from build123d import *

# Parameters (mm, degrees)
F1_DEPTH = 50
F1_TAPER = -3
F2_R     = 35
F3_SIZE  = 10
F5_DEPTH = 10


with BuildPart() as f1:
    # F0 (on Top) → F1 (new body)
    with BuildSketch(Plane.XY):
        with BuildLine():
            ThreePointArc((150, -150), (300, 0), (150, 150))
            Line((150, 150), (-150, 150))
            ThreePointArc((-150, 150), (-300, 0), (-150, -150))
            Line((-150, -150), (150, -150))
        make_face()
    extrude(amount=F1_DEPTH, taper=F1_TAPER)

    # F2
    f2_edges = [f1.edges().sort_by_distance(p)[0] for p in [
        (-302.620389, 0, 50),
        (0, -152.620389, 50),
        (302.620389, 0, 50),
        (0, 152.620389, 50),
    ]]
    fillet(f2_edges, radius=F2_R)

    # F3
    f3_edges = [f1.edges().sort_by_distance(p)[0] for p in [
        (-300, 0, 0),
        (0, -150, 0),
        (300, 0, 0),
        (0, 150, 0),
    ]]
    chamfer(f3_edges, length=F3_SIZE)

    # F4 (on face) → F5 (join)
    with BuildSketch(Plane(origin=(0, 0, 0), x_dir=(1, 0, 0), z_dir=(0, 0, -1))):
        with BuildLine():
            Line((150, 128), (-150, 128))
            ThreePointArc((-150, 128), (-278, 0), (-150, -128))
            Line((-150, -128), (150, -128))
            ThreePointArc((150, -128), (278, 0), (150, 128))
        make_face()
    extrude(amount=F5_DEPTH)


solid = f1.part
Read the model definition and answer for the solid it produces. Units are mm, in the model's axes. A direction names the side the tool comes from. Give positions to 0.01 mm unless a question says otherwise; leave off trailing zeros. Loops run counter-clockwise (first coordinate to the right, second up) from the corner with the lowest first, then second, coordinate; pieces in that order, holes last. Notation, with made-up numbers: (39.25, 64.5) - (65.25, 64.5) arc R9 ccw to (65.25, 81.5) - close; hole circle Ø5 at (74.25, -5). An arc over 180 degrees is marked (long way). Answer as CSV lines item,"result". Start each with the question number.
1) Find section B-B (z = 27.5). Write down the section's boundary in (x, y), then the cut area to 3 significant figures.
2) Find section A-A (x = 100). Write down the section's boundary in (y, z), then the cut area to 3 significant figures.
3) Which of the six approach directions +Z, -Z, +X, -X, +Y, -Y give full straight-line access (tool end or side, diameter ignored) to faces 1 (the face through (1, -134, 0)), 2 (the face through (-4, -2, -10)), 3 (the face through (-277.97, -2.81, -4.93)), 4 (the face through (277.97, 2.81, -4.93))?
4) Each of these flat-tipped pins is pushed along its axis until it touches: pin 1 Ø2 at (y, z) = (72.5, 25) entering from -X; pin 2 Ø1.5 at (x, z) = (-214, 10.5) entering from +Y; pin 3 Ø3 at (y, z) = (-6, 25) entering from +X. Where does it stop, or does it pass through?
5) Straight lines are drawn through the part: L1, parallel to Y at x = -108.5, z = 22; L2, parallel to Y at x = 2.5, z = -1.5; L3, parallel to X at y = -96, z = -1.5. For each, find the intervals that lie inside material, in ascending order. Write a range as from..to.
Findings below:
1,outline,"(-150, -148.43) - (150, -148.43) arc R148.43 ccw to (150, 148.43) - (-150, 148.43) arc R148.43 ccw to start"
1,area,"158,000 mm^2"
2,outline,"(-150.69, 13.17) - (-150.52, 9.99) - (-140, 0) - (-128, 0) - (-128, -10) - (128, -10) - (128, 0) - (140, 0) - (150.52, 9.99) - (150.69, 13.17) arc R35 ccw to (115.74, 50) - (-115.74, 50) arc R35 ccw to start"
2,area,"17,000 mm^2"
3,face 1,"-Z"
3,face 2,"-Z, +X, -X, +Y, -Y"
3,face 3,"-Z, -X"
3,face 4,"-Z, +X"
4,pin 1,"x = -281.13"
4,pin 2,"y = 136.62"
4,pin 3,"x = 299.57"
5,L1,"-150.03..150.03"
5,L2,"-128..128"
5,L3,"-234.66..234.66"
